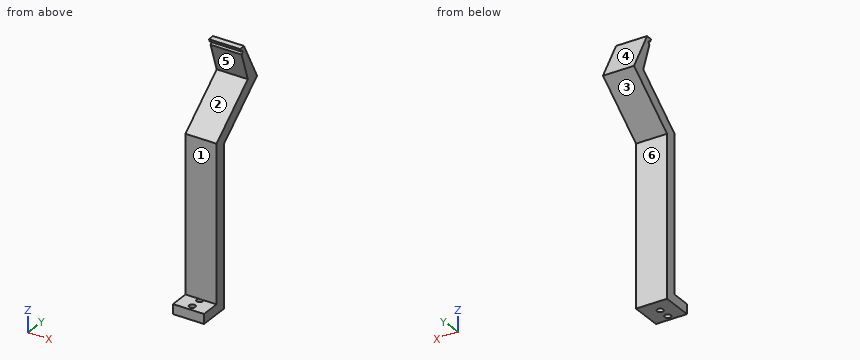
Autodesk Inventor part; units mm, degrees
ref_plane "YZ Plane" through (0, 0, 0) normal (1, 0, 0) x (0, 1, 0)
ref_plane "XZ Plane" through (0, 0, 0) normal (0, 1, 0) x (-1, 0, 0)
ref_plane "XY Plane" through (0, 0, 0) normal (0, 0, 1) x (1, 0, 0)
ref_plane "Arbeitsebene1" through (0, 10.2818, 0) normal (0, 0, 1) x (1, 0, 0)
sketch "Skizze1" plane through (0, 10.2818, 0) normal (0, 0, 1) x (1, 0, 0)
  circle A0 centre (10, 10.7182) radius 1.4
  circle A1 centre (10, 4.7182) radius 1.4
  circle A2 centre (10, -1.2818) radius 1.4
  circle A3 centre (10, -7.2818) radius 1.4
  line L0 (0, 12.7182) -> (2, 14.7182)
  line L1 (0, -8.2818) -> (0, 12.7182)
  line L2 (2, -10.2818) -> (0, -8.2818)
  line L3 (2, -10.2818) -> (18, -10.2818)
  line L4 (20, -8.2818) -> (18, -10.2818)
  line L5 (20, -8.2818) -> (20, 12.7182)
  line L6 (18, 14.7182) -> (20, 12.7182)
  line L7 (2, 14.7182) -> (18, 14.7182)
  line L8 (18, -10.2818) -> (2, -10.2818)
  line L9 (2, -10.2818) -> (2, 5.7182)
  line L10 (2, 5.7182) -> (18, 5.7182)
  line L11 (18, 5.7182) -> (18, -10.2818)
  circle A4 centre (10, -1.2818) radius 1.6
  circle A5 centre (10, -7.2818) radius 1.6
  point P0 (0, -10.2818)
  point P1 (2, -10.2818)
  dimension "d0" = 16
  dimension "d1" = 3.2
  dimension "d2" = 3.2
extrude "Extrusion1" add sketch "Skizze1" along normal blind 5 contours A1 L10 | A1 L10 L11 L3 L9 picked at (10.1558, 4.945)
sketch "Skizze2" plane through (18, 0, 0) normal (1, 0, 0) x (0, 0, -1)
  line L0 (0, 0) -> (0, 16)
  line L1 (0, 16) -> (-5, 16)
  line L2 (-5, 0) -> (-5, 16)
  line L3 (0, 0) -> (-5, 0)
  line L4 (-5, 16) -> (100, 16) construction
  line L5 (-103.3677, 42.3666) -> (-123.2187, 31.877)
  line L6 (-123.2187, 31.877) -> (-123.0578, 28.8814)
  line L7 (-123.0578, 28.8814) -> (-105.1383, 35)
  line L8 (-5, 10) -> (-85, 10)
  line L9 (-85, 10) -> (-105.1383, 35)
  line L10 (-5, 16) -> (-82.1287, 16)
  line L11 (-82.1287, 16) -> (-103.3677, 42.3666)
  point P0 (0, 0)
  point P1 (-123.1383, 30.3792)
  dimension "d8" = 3
  dimension "d9" = 6
  dimension "d15" = 80
  dimension "d16" = 6
  dimension "d17" = 9
  dimension "d18" = 110
  dimension "d19" = 18
  dimension "d20" = 25
extrude "Extrusion2" add sketch "Skizze2" against normal up to surface (16 mm away) contours L2 L8 L9 L7 L6 L5 L11 L10
sketch "Skizze3" plane through (18, 0, 0) normal (1, 0, 0) x (0, 0, -1)
  line L0 (0, 0) -> (0, 16)
  line L1 (0, 16) -> (-82.1287, 16)
  line L2 (-103.3677, 42.3666) -> (-123.2187, 31.877)
  line L3 (-123.2187, 31.877) -> (-123.0578, 28.8814)
  line L4 (-123.0578, 28.8814) -> (-105.1383, 35)
  line L5 (-5, 0) -> (-5, 10)
  line L6 (0, 0) -> (-5, 0)
  circle A0 centre (-120.723, 29.6786) radius 1
  line L7 (-82.1287, 16) -> (-103.3677, 42.3666)
  line L8 (-105.1383, 35) -> (-85, 10)
  line L9 (-85, 10) -> (-5, 10)
  point P0 (0, 0)
  point P1 (-119.7766, 30.0017)
  point P2 (-121.6693, 29.3555)
  dimension "d12" = 2
extrude "Extrusion3" cut sketch "Skizze3" against normal through all contours L4 A0 picked at (-121.0524, 29.7298)
properties part number "OT2-Gripper_finger"
Could you check a few things on this model? Use its own coordinates, in mm. Face numbers are marked on the shaded views. A direction names the side the tool comes from. Round coordinates to 2 decimals unless told otherwise and drop trailing zeros. Loops run counter-clockwise (first coordinate to the right, second up) from the corner with the lowest first, then second, coordinate; pieces in that order, holes last.
Q1. Thinking about a two-plate mould opening in Z: for the marked faces 4, 5 and 6, which applies, pulls with the +Z half, pulls with the -Z half, needs draft (parallel to the pull), parting line crosses it, or undercut?
Q2. For P1, Ø8, axis at x = 8, z = 51, coming from the +Y side; P2, Ø1.5, axis at x = 15.5, z = 43.5, coming from the -Y side; P3, Ø1.9, axis at x = 10, y = 9, coming from the +Z side; P4, Ø5, axis at x = 6, z = 83.5, coming from the +Y side, each with a flat end and sliding along its axis, tell me the tip position at first contact or that it passes through.
Q3. I want a section at B-B (z = 10.5). Write out the boundary of the cut face in (x, y).
Q4. On a 3-axis mill with a long thin cutter (end or side, diameter ignored), from which of +Z, -Z, +X, -X, +Y, -Y can I reach the whole of each face in a straight line? I mean the marked faces 1, 2 and 3. Say none if no direction works.
Q5. Please list where these lines run through material, in increasing order: L1, parallel to Y at x = 10, z = 3.4; L2, parallel to X at y = 9, z = 2.2; L3, parallel to Y at x = 7.25, z = 29.5.
Q6. I want a section at C-C (y = 21.5). Write out the boundary of the cut face in (x, z), and give its area (3 significant figures).
Q7. I want a section at A-A (x = 10). Write out the boundary of the cut face in (y, z).
Answer below:
1. face 4: pulls with the +Z half
1. face 5: undercut
1. face 6: needs draft
2. P1: stops at y = 16
2. P2: stops at y = 10
2. P3: passes through
2. P4: stops at y = 20.81
3. outline: (2, 10) - (18, 10) - (18, 16) - (2, 16) - close
4. face 1: +Z, +X, -X, -Y
4. face 2: +X, -X, -Y
4. face 3: -Z, +X, -X, +Y
5. L1: y = 0 to 1.4, 4.6 to 7.4, 10.6 to 16
5. L2: x = 2 to 8.4, 11.6 to 18
5. L3: y = 10 to 16
6. outline: (2, 86.56) - (18, 86.56) - (18, 94.26) - (2, 94.26) - close
6. area: 123 mm2
7. outline: (0, 0) - (1.4, 0) - (1.4, 5) - (0, 5) - close; (4.6, 0) - (7.4, 0) - (7.4, 5) - (4.6, 5) - close; (10, 5) - (10.6, 5) - (10.6, 0) - (16, 0) - (16, 82.13) - (42.37, 103.37) - (31.88, 123.22) - (28.88, 123.06) - (29.36, 121.67) arc R1 cw to (30, 119.78) - (35, 105.14) - (10, 85) - close
